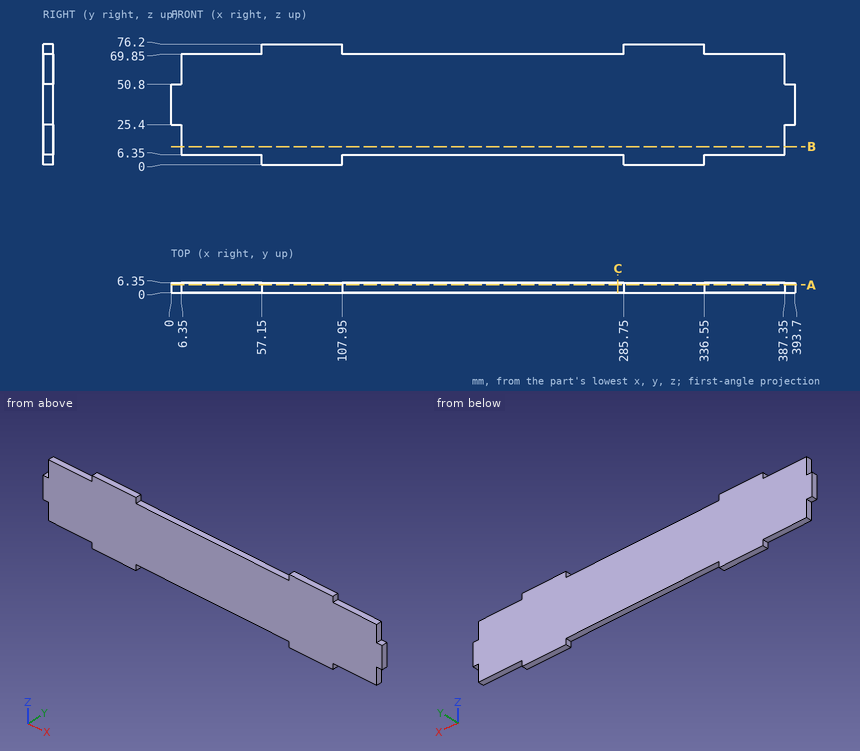
Geometry: see drawing. Coordinates: mm, zero at the bounding-box minimum. Round coordinates to 2 decimals unless told otherwise and drop trailing zeros. Write each loop counter-clockwise with the first axis right and the second up, starting at its lowest first coordinate (ties: lowest second). Pieces come first, ordered by that corner, then holes. Notation, with made-up numbers: M 77.5,-16 L 89.5,-16 A34 cw 89.5,21 Z; hole C 37,-28.75 d1. An arc over 180 degrees is marked long. Answer in a Markdown table with one row per item. Add a question column.
(1) Cut plane A-A, the plane y = 5. Return the cut outline in (x, z).
(2) Contact query for flat-ended pins moving along their axis: pin 1 (1.9 mm diameter, centred on y = 2, z = 2, fed in from -X); pin 2 (3 mm diameter, centred on y = 3.5, z = 11.5, fed in from -X); pin 3 (1.9 mm diameter, centred on x = 361, y = 2.5, fed in from +Z). Output: stop coordinate, or through.
(3) Cut plane C-C, the plane x = 282. Return the cut outline in (y, z), then the cut area to 3 significant figures.
(4) Ray query, L1, parallel to X at y = 1.25, z = 70; L2, parallel to Z at x = 176, y = 1; L3, parallel to X at y = 4, z = 14.5. Return the intervals inside material, ascending.
(5) Cut plane B-B, the plane z = 11.5. Return the cut outline in (x, y), then the cut area to 3 significant figures.
Established:
| question | item | result |
|---|---|---|
| 1 | outline | M 0,25.4 L 6.35,25.4 L 6.35,6.35 L 57.15,6.35 L 57.15,0 L 107.95,0 L 107.95,6.35 L 285.75,6.35 L 285.75,0 L 336.55,0 L 336.55,6.35 L 387.35,6.35 L 387.35,25.4 L 393.7,25.4 L 393.7,50.8 L 387.35,50.8 L 387.35,69.85 L 336.55,69.85 L 336.55,76.2 L 285.75,76.2 L 285.75,69.85 L 107.95,69.85 L 107.95,76.2 L 57.15,76.2 L 57.15,69.85 L 6.35,69.85 L 6.35,50.8 L 0,50.8 Z |
| 2 | pin 1 | x = 57.15 |
| 2 | pin 2 | x = 6.35 |
| 2 | pin 3 | z = 69.85 |
| 3 | outline | M 0,6.35 L 6.35,6.35 L 6.35,69.85 L 0,69.85 Z |
| 3 | area | 403 mm² |
| 4 | L1 | 57.15 to 107.95, 285.75 to 336.55 |
| 4 | L2 | 6.35 to 69.85 |
| 4 | L3 | 6.35 to 387.35 |
| 5 | outline | M 6.35,0 L 387.35,0 L 387.35,6.35 L 6.35,6.35 Z |
| 5 | area | 2,420 mm² |
